from build123d import *

# Parameters (mm, degrees)
F0_W     = 88.9
F0_H     = 38.1
F1_DEPTH = 1524
F2_W     = 38.1
F2_H     = 50.8
F3_DEPTH = 38.1
F4_W     = 38.1
F4_H     = 63.5
F5_DEPTH = 38.1


with BuildPart() as f1:
    # F0 (on Top) → F1 (new body)
    with BuildSketch(Plane.XY):
        with Locations((44.45, 19.05)):
            Rectangle(F0_W, F0_H)
    extrude(amount=F1_DEPTH)

    # F2 (on face) → F3 (cut, through all)
    with BuildSketch(Plane(origin=(0, 38.1, 0), x_dir=(-1, 0, 0), z_dir=(0, 1, 0))):
        with Locations((-44.45, 1092.2)):
            Rectangle(F2_W, F2_H)
    extrude(amount=-F3_DEPTH, mode=Mode.SUBTRACT)

    # F4 (on face) → F5 (cut, through all)
    with BuildSketch(Plane.XZ):
        with Locations((44.45, 539.75)):
            Rectangle(F4_W, F4_H)
    extrude(amount=-F5_DEPTH, mode=Mode.SUBTRACT)


solid = f1.part
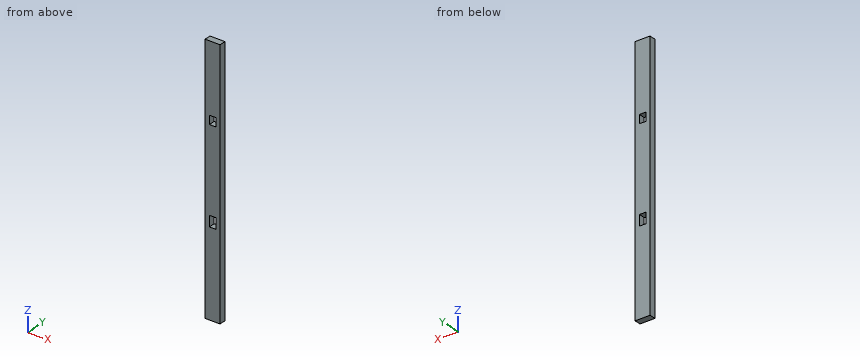
Read the model definition and answer for the solid it produces. Units are mm, in the model's axes. Coordinates: 2 decimals unless noted, no trailing zeros. Write each loop counter-clockwise with the first axis right and the second up, starting at its lowest first coordinate (ties: lowest second). Pieces come first, ordered by that corner, then holes. Notation, with made-up numbers: M 25.5,12 L 29.5,12 A29 cw 29.5,38 Z; hole C 12.25,1.5 d11. An arc over 180 degrees is marked long. Use a Markdown table: item, result.
Q1. The part is cut by section C-C, the plane x = 41.5. Write down the section's boundary in (y, z), then the cut area to 3 significant figures.
Answer block:
| item | result |
|---|---|
| outline | M 0,0 L 38.1,0 L 38.1,508 L 0,508 Z; M 0,571.5 L 38.1,571.5 L 38.1,1066.8 L 0,1066.8 Z; M 0,1117.6 L 38.1,1117.6 L 38.1,1524 L 0,1524 Z |
| area | 53,700 mm2 |
Q2. The part is cut by section A-A, the plane z = 543.5. Write down the section's boundary in (x, y).
Answer block:
| item | result |
|---|---|
| outline | M 0,0 L 25.4,0 L 25.4,38.1 L 0,38.1 Z; M 63.5,0 L 88.9,0 L 88.9,38.1 L 63.5,38.1 Z |
Q3. A straight line is drawn through the part: L1, parallel to Z at x = 44.5, y = 24.5. Find the intervals that lie inside material, in ascending order. Write a range as [from, to].
Answer block:
| item | result |
|---|---|
| L1 | z = [0, 508], [571.5, 1066.8], [1117.6, 1524] |
Q4. The part is cut by section B-B, the plane y = 15. Write down the section's boundary in (x, z).
Answer block:
| item | result |
|---|---|
| outline | M 0,0 L 88.9,0 L 88.9,1524 L 0,1524 Z; hole M 25.4,508 L 63.5,508 L 63.5,571.5 L 25.4,571.5 Z; hole M 25.4,1066.8 L 63.5,1066.8 L 63.5,1117.6 L 25.4,1117.6 Z |
